Here's how the part is built. I have some questions about the finished solid (model axes, mm). Face numbers are marked on the shaded views. A direction names the side the tool comes from. Round coordinates to 2 decimals unless told otherwise and drop trailing zeros. Order: outer loops, then holes, each group sorted by start corner. A loop starts at its lowest first (then second) coordinate and runs counter-clockwise, first axis right, second up. Notation, with made-up numbers: (-8.5, 70) -> (24.5, 70) arc R20 cw to (24.5, 90) -> close; hole circle Ø1 at (-5.5, -22.5). An arc over 180 degrees is marked (long way). Use a Markdown table: item, result. Add a question column.
(1) I want a section at C-C, the plane z = -10. Please give me the cut outline in (x, y).
(2) On a 3-axis mill with a long thin cutter (end or side, diameter ignored), from which of +Z, -Z, +X, -X, +Y, -Y can I reach the whole of each face in a straight line? I mean the marked faces 4, 5, 6, 7 and 8. Say none if no direction works.
(3) I'm going to push flat-ended pins straight in: P1, Ø0.5, axis at x = 18, y = 7, coming from the +Z side; P2, Ø1.6, axis at x = 8.66, z = -5, coming from the -Y side; P3, Ø1, axis at x = 6.5, y = 5.5, coming from the -Z side. Where does each tip first touch, or does it pass through?
(4) If I drill on probe 1 along Z at (x, y) = (0, 4.05); probe 2 along X at (y, z) = (4.75, -5) (3 decimals); probe 3 along X at (y, z) = (7.5, 3.25), over which ranges is the centre line in solid material (lowest first)?
(5) I want a section at D-D, the plane x = 18. Please give me the cut outline in (y, z).
(6) Thinking about a two-plate mould opening in X: for the marked faces 1, 2 and 3, which applies, pulls with the +X half, pulls with the -X half, needs draft (parallel to the pull), parting line crosses it, or undercut?
(7) I want a section at A-A, the plane z = 0. Please give me the cut outline in (x, y), then the cut area to 3 significant figures.
(8) I want a section at B-B, the plane x = 25. Please give me the cut outline in (y, z).
from build123d import *

# Parameters (mm, degrees)
SKETCH_1_R          = 13.5
SKETCH_1_R_2        = 1.6
EXTRUDE_1_DEPTH     = 10
EXTRUDE_START       = -6
SKETCH_2_R          = 1
EXTRUDE_2_DEPTH     = 6
SKETCH_3_R          = 3
CUT_EXTRUDE_1_DEPTH = 5
SKETCH_4_R          = 3
SKETCH_4_R_2        = 1
EXTRUDE_3_DEPTH     = 0.7
FILLET_1_R          = 10
FILLET_2_R          = 2
HOLE_WIZARD_M3_1_D  = 2.5
F_2_0MM_2_D         = 2
F_2_0MM_2_DEPTH     = 6
F_2_0MM_2_TIP       = 0.600860619


with BuildPart() as part:
    # 草图1 → 凸台-拉伸1 (new body)
    with BuildSketch(Plane(origin=(0, 0, 0), x_dir=(1, 0, 0), z_dir=(0, 1, 0))):
        with Locations(Location((0, 0, 0), (0, 0, 270))):
            Circle(SKETCH_1_R)
        with Locations(Location((0, 10, 0), (0, 0, 270))):
            Circle(SKETCH_1_R_2, mode=Mode.SUBTRACT)
        with Locations(Location((8.660254038, -5, 0), (0, 0, 270))):
            Circle(SKETCH_1_R_2, mode=Mode.SUBTRACT)
        with Locations(Location((-8.660254038, -5, 0), (0, 0, 270))):
            Circle(SKETCH_1_R_2, mode=Mode.SUBTRACT)
    extrude(amount=EXTRUDE_1_DEPTH)

    # 草图2 → 凸台-拉伸2 (add)
    # profile 1 of 2: a face of its own
    with BuildSketch(Plane(origin=(0, 10, 0), x_dir=(1, 0, 0), z_dir=(0, 1, 0)).offset(EXTRUDE_START)):
        with BuildLine():
            Line((-12.093386622, 6), (-19.708497378, 6))
            ThreePointArc((-19.708497378, 6), (-33, 0), (-19.708497378, -6))
            Line((-19.708497378, -6), (-12.093386622, -6))
            ThreePointArc((-12.093386622, -6), (-13.5, 0), (-12.093386622, 6))
        make_face()
        with Locations(Location((-25, 0, 0), (0, 0, 270))):
            Circle(SKETCH_2_R, mode=Mode.SUBTRACT)
    # profile 2 of 2: a face of its own
    with BuildSketch(Plane(origin=(0, 10, 0), x_dir=(1, 0, 0), z_dir=(0, 1, 0)).offset(EXTRUDE_START)):
        with BuildLine():
            ThreePointArc((13.5, 0), (13.143643319, -3.08133742), (12.093386622, -6))
            Line((12.093386622, -6), (19.708497378, -6))
            ThreePointArc((19.708497378, -6), (33, 0), (19.708497378, 6))
            Line((19.708497378, 6), (12.093386622, 6))
            ThreePointArc((12.093386622, 6), (13.143643319, 3.08133742), (13.5, 0))
        make_face()
        with Locations(Location((25, 0, 0), (0, 0, 270))):
            Circle(SKETCH_2_R, mode=Mode.SUBTRACT)
    extrude(amount=EXTRUDE_2_DEPTH)

    # 草图3 → 切除-拉伸1 (cut)
    with BuildSketch(Plane(origin=(0, 10, 0), x_dir=(1, 0, 0), z_dir=(0, 1, 0))):
        with Locations(Location((0, 10, 0), (0, 0, 270))):
            Circle(SKETCH_3_R)
        with Locations(Location((8.660254038, -5, 0), (0, 0, 270))):
            Circle(SKETCH_3_R)
        with Locations(Location((-8.660254038, -5, 0), (0, 0, 270))):
            Circle(SKETCH_3_R)
    extrude(amount=-CUT_EXTRUDE_1_DEPTH, mode=Mode.SUBTRACT)

    # 草图4 → 凸台-拉伸3 (add)
    # profile 1 of 2: a face of its own
    with BuildSketch(Plane(origin=(0, 10, 0), x_dir=(1, 0, 0), z_dir=(0, 1, 0))):
        with Locations(Location((-25, 0, 0), (0, 0, 270))):
            Circle(SKETCH_4_R)
        with Locations(Location((-25, 0, 0), (0, 0, 270))):
            Circle(SKETCH_4_R_2, mode=Mode.SUBTRACT)
    # profile 2 of 2: a face of its own
    with BuildSketch(Plane(origin=(0, 10, 0), x_dir=(1, 0, 0), z_dir=(0, 1, 0))):
        with Locations(Location((25, 0, 0), (0, 0, 270))):
            Circle(SKETCH_4_R)
        with Locations(Location((25, 0, 0), (0, 0, 270))):
            Circle(SKETCH_4_R_2, mode=Mode.SUBTRACT)
    extrude(amount=EXTRUDE_3_DEPTH)

    # 圆角1
    fillet_1_edges = [part.edges().sort_by_distance(p)[0] for p in [
        (-12.093386622, 7, -6),
        (-12.093386622, 7, 6),
        (12.093386622, 7, 6),
        (12.093386622, 7, -6),
    ]]
    fillet(fillet_1_edges, radius=FILLET_1_R)

    # 圆角2
    fillet_2_edges = [part.edges().sort_by_distance(p)[0] for p in [
        (-19.708497378, 7, -6),
        (-19.708497378, 7, 6),
        (19.708497378, 7, -6),
        (19.708497378, 7, 6),
    ]]
    fillet(fillet_2_edges, radius=FILLET_2_R)

    # M3 螺纹孔1 (through all)
    with Locations(Plane(origin=(0, 10.7, 0), x_dir=(1, 0, 0), z_dir=(0, 1, 0))):
        with Locations((-25, 0), (25, 0)):
            Hole(HOLE_WIZARD_M3_1_D / 2)

    # Ø2.0mm 暗销孔2
    with Locations(Plane.XZ):
        with Locations((-8.660254038, -5), (0, 10), (8.660254038, -5)):
            Hole(F_2_0MM_2_D / 2, depth=F_2_0MM_2_DEPTH)
            with Locations((0, 0, -(F_2_0MM_2_DEPTH + F_2_0MM_2_TIP / 2))):  # 118° drill point
                Cone(0, F_2_0MM_2_D / 2, F_2_0MM_2_TIP, mode=Mode.SUBTRACT)


solid = part.part
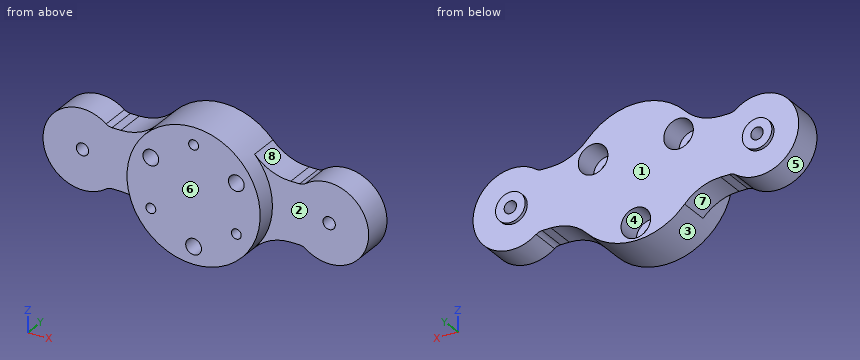
Taken from the geometry:
| question | item | result |
|---|---|---|
| 1 | outline | (-9.07, 0) -> (-1.6, 0) -> (-1.6, 5) -> (-3, 5) -> (-3, 10) -> (-9.07, 10) -> close; (1.6, 0) -> (9.07, 0) -> (9.07, 10) -> (3, 10) -> (3, 5) -> (1.6, 5) -> close |
| 2 | face 4 | +Y |
| 2 | face 5 | +Y, -Y |
| 2 | face 6 | +Z, -Z, +X, -X, -Y |
| 2 | face 7 | -Z, +Y, -Y |
| 2 | face 8 | +Z, +Y, -Y |
| 3 | P1 | stops at z = 6 |
| 3 | P2 | stops at y = 6.12 |
| 3 | P3 | stops at z = -12.09 |
| 4 | probe 1 | z = -13.5 to -11.6, -8.4 to 9, 11 to 13.5 |
| 4 | probe 2 | x = -31.245 to -9.66, -7.66 to 7.66, 9.66 to 31.245 |
| 4 | probe 3 | x = -32.31 to -11.1, -6.22 to 6.22, 11.1 to 32.31 |
| 5 | outline | (4, -6) -> (10, -6) -> (10, 6) -> (4, 6) -> close |
| 6 | face 1 | undercut |
| 6 | face 2 | needs draft |
| 6 | face 3 | parting line crosses it |
| 7 | outline | (-33, 4) -> (-26.25, 4) -> (-26.25, 10.7) -> (-28, 10.7) -> (-28, 10) -> (-33, 10) -> close; (-23.75, 4) -> (-13.5, 4) -> (-13.5, 0) -> (13.5, 0) -> (13.5, 4) -> (23.75, 4) -> (23.75, 10.7) -> (22, 10.7) -> (22, 10) -> (-22, 10) -> (-22, 10.7) -> (-23.75, 10.7) -> close; (26.25, 4) -> (33, 4) -> (33, 10) -> (28, 10) -> (28, 10.7) -> (26.25, 10.7) -> close |
| 7 | area | 479 mm2 |
| 8 | outline | (4, -8) -> (10, -8) -> (10, -3) -> (10.7, -3) -> (10.7, -1.25) -> (4, -1.25) -> close; (4, 1.25) -> (10.7, 1.25) -> (10.7, 3) -> (10, 3) -> (10, 8) -> (4, 8) -> close |
